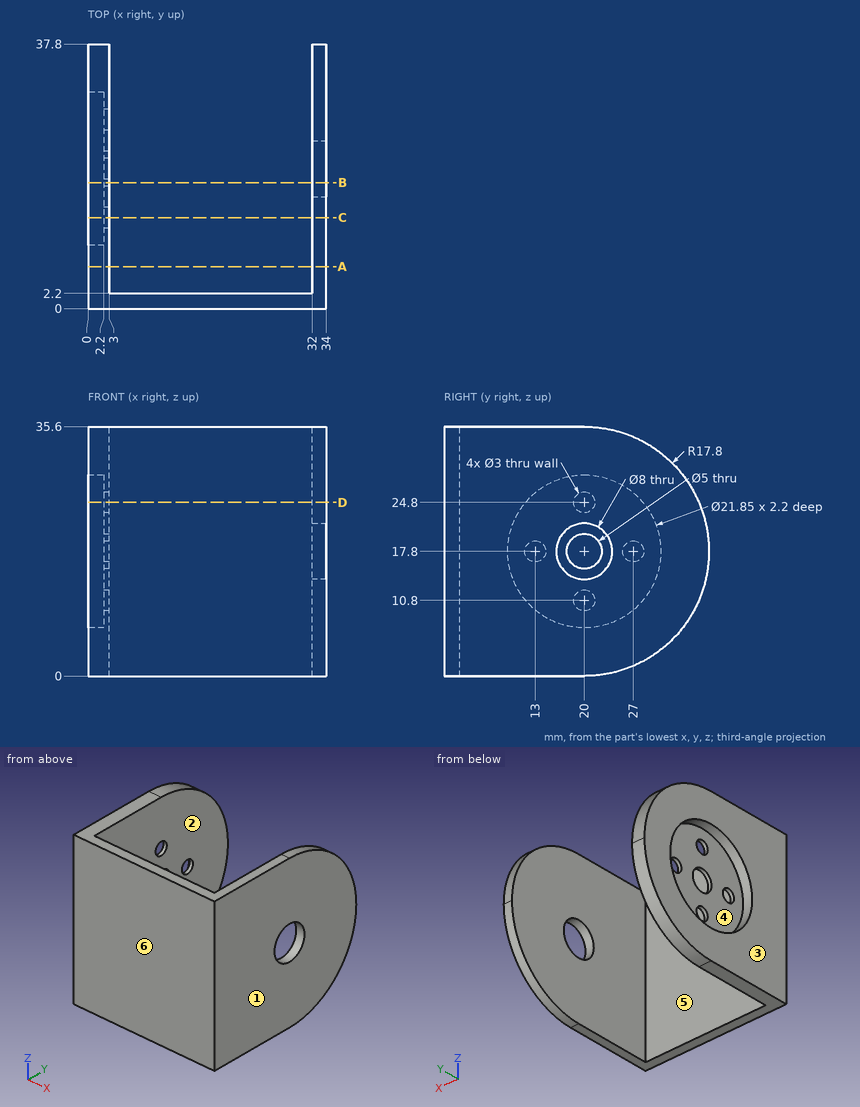
The drawing under review shows one solid part. Ordinate dimensions are in mm from its lowest x, y, z. A direction names the side the tool comes from. Give positions to 0.01 mm unless a question says otherwise; leave off trailing zeros. Write each loop counter-clockwise with the first axis right and the second up, starting at its lowest first coordinate (ties: lowest second). Pieces come first, ordered by that corner, then holes. Notation, with made-up numbers: (37.25, 47) -> (80.25, 47) arc R16 ccw to (80.25, 54) -> close; hole circle Ø9 at (-11, 4). An arc over 180 degrees is marked (long way). Answer in a Markdown table with one row per item.
(1) Consider section C-C (y = 13). State the section outline as (x, z) points, then the cut area to 3 significant figures.
Results:
| item | result |
|---|---|
| outline | (0, 0) -> (3, 0) -> (3, 16.3) -> (2.2, 16.3) -> (2.2, 9.41) -> (0, 9.41) -> close; (0, 26.19) -> (2.2, 26.19) -> (2.2, 19.3) -> (3, 19.3) -> (3, 35.6) -> (0, 35.6) -> close; (32, 0) -> (34, 0) -> (34, 35.6) -> (32, 35.6) -> close |
| area | 139 mm2 |
(2) Clearance check with flat-ended pins moving along their axes: pin 1 (19.5 mm diameter, centred on y = 20, z = 17.8, fed in from -X); pin 2 (2 mm diameter, centred on x = 16.5, z = 21, fed in from +Y); pin 3 (1.8 mm diameter, centred on y = 27, z = 17.8, fed in from -X); pin 4 (3 mm diameter, centred on x = 29, y = 15, fed in from +Z). State where each tip first meets the part, or that it passes through.
Results:
| item | result |
|---|---|
| pin 1 | x = 2.2 |
| pin 2 | y = 2.2 |
| pin 3 | x = 32 |
| pin 4 | through |
(3) Consider section A-A (y = 6). State the section outline as (x, z) points.
Results:
| item | result |
|---|---|
| outline | (0, 0) -> (3, 0) -> (3, 35.6) -> (0, 35.6) -> close; (32, 0) -> (34, 0) -> (34, 35.6) -> (32, 35.6) -> close |
(4) For the marked faces 4, 5 and 6, list the 3-axis set-ups (+Z, -Z, +X, -X, +Y, -Y) from which the entire face can be reached by the end or side of a thin tool; tool diameter is ignored.
Results:
| item | result |
|---|---|
| face 4 | -X |
| face 5 | +Z, -Z, +Y |
| face 6 | +Z, -Z, +X, -X, -Y |
(5) Consider section B-B (y = 18). State the section outline as (x, z) points.
Results:
| item | result |
|---|---|
| outline | (0, 0) -> (3, 0) -> (3, 16.3) -> (2.2, 16.3) -> (2.2, 7.06) -> (0, 7.06) -> close; (0, 28.54) -> (2.2, 28.54) -> (2.2, 19.3) -> (3, 19.3) -> (3, 35.6) -> (0, 35.6) -> close; (32, 0) -> (34, 0) -> (34, 14.34) -> (32, 14.34) -> close; (32, 21.26) -> (34, 21.26) -> (34, 35.6) -> (32, 35.6) -> close |
(6) Mouldability with a two-part tool opening along X and no side actions: class the marked faces 1, 2 and 3 as +X half, -X half, draft (parallel to the pull), parting line (faces both ways), or undercut.
Results:
| item | result |
|---|---|
| face 1 | +X half |
| face 2 | undercut |
| face 3 | -X half |
(7) To check wall thickness, follow probe 1 along Y at (x, z) = (2.85, 17.8); probe 2 along X at (y, z) = (23, 22.5); probe 3 along X at (y, z) = (35, 21.5). State the ranges of each line that lie inside material, in increasing order.
Results:
| item | result |
|---|---|
| probe 1 | 0 to 11.5, 14.5 to 17.5, 22.5 to 25.5, 28.5 to 37.8 |
| probe 2 | 2.2 to 3, 32 to 34 |
| probe 3 | 0 to 3, 32 to 34 |
(8) Consider section D-D (z = 24.8). State the section outline as (x, y) points.
Results:
| item | result |
|---|---|
| outline | (0, 0) -> (34, 0) -> (34, 36.37) -> (32, 36.37) -> (32, 2.2) -> (3, 2.2) -> (3, 18.5) -> (2.2, 18.5) -> (2.2, 11.61) -> (0, 11.61) -> close; (0, 28.39) -> (2.2, 28.39) -> (2.2, 21.5) -> (3, 21.5) -> (3, 36.37) -> (0, 36.37) -> close |
